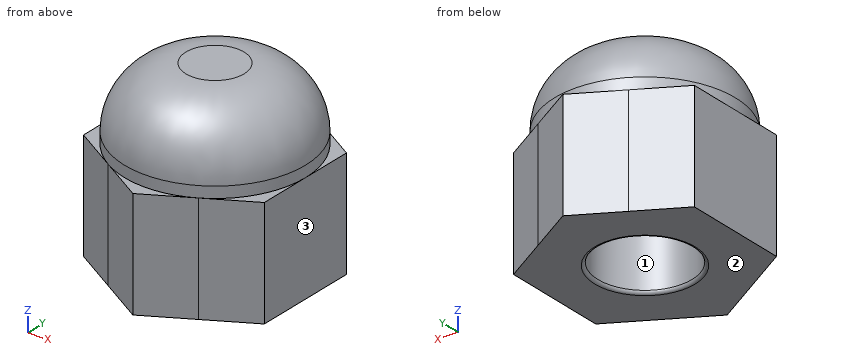
from build123d import *

# Parameters (mm, degrees)
SKETCH1_R           = 7.5
SKETCH1_R_2         = 3.9
BOSS_EXTRUDE1_DEPTH = 9
SKETCH2_R           = 7.5
BOSS_EXTRUDE2_DEPTH = 6
FILLET1_R           = 5.08
FILLET2_R           = 0.254


with BuildPart() as part:
    # Sketch1 → Boss-Extrude1 (new body)
    # profile 1 of 7: a face of its own
    with BuildSketch(Plane(origin=(0, 0, 0), x_dir=(0, 1, 0), z_dir=(0, 0, 1))):
        with BuildLine():
            ThreePointArc((-6.495190512, 3.750000029), (-3.749999976, 6.495190542), (2.2e-08, 7.5))
            Line((2.2e-08, 7.5), (-4.330127019, 7.5))
            Line((-4.330127019, 7.5), (-6.495190512, 3.750000029))
        make_face()
    # profile 2 of 7: a face of its own
    with BuildSketch(Plane(origin=(0, 0, 0), x_dir=(0, 1, 0), z_dir=(0, 0, 1))):
        Circle(SKETCH1_R)
        with Locations(Location((0, 0, 0), (0, 0, 270))):
            Circle(SKETCH1_R_2, mode=Mode.SUBTRACT)
    # profile 3 of 7: a face of its own
    with BuildSketch(Plane(origin=(0, 0, 0), x_dir=(0, 1, 0), z_dir=(0, 0, 1))):
        with BuildLine():
            ThreePointArc((2.2e-08, 7.5), (3.749999991, 6.495190533), (6.495190507, 3.750000037))
            Line((6.495190507, 3.750000037), (4.330127019, 7.5))
            Line((4.330127019, 7.5), (2.2e-08, 7.5))
        make_face()
    # profile 4 of 7: a face of its own
    with BuildSketch(Plane(origin=(0, 0, 0), x_dir=(0, 1, 0), z_dir=(0, 0, 1))):
        with BuildLine():
            ThreePointArc((-6.495190559, -3.749999947), (-7.5, 4.7e-08), (-6.495190512, 3.750000029))
            Line((-6.495190512, 3.750000029), (-8.660254038, 0))
            Line((-8.660254038, 0), (-6.495190559, -3.749999947))
        make_face()
    # profile 5 of 7: a face of its own
    with BuildSketch(Plane(origin=(0, 0, 0), x_dir=(0, 1, 0), z_dir=(0, 0, 1))):
        with BuildLine():
            Line((6.49519047, -3.750000102), (8.660254038, 0))
            Line((8.660254038, 0), (6.495190507, 3.750000037))
            ThreePointArc((6.495190507, 3.750000037), (7.244443692, 1.941142859), (7.5, 0))
            ThreePointArc((7.5, 0), (7.244443682, -1.941142895), (6.49519047, -3.750000102))
        make_face()
    # profile 6 of 7: a face of its own
    with BuildSketch(Plane(origin=(0, 0, 0), x_dir=(0, 1, 0), z_dir=(0, 0, 1))):
        with BuildLine():
            Line((4.330127019, -7.5), (6.49519047, -3.750000102))
            ThreePointArc((6.49519047, -3.750000102), (3.749999939, -6.495190564), (-2.3e-08, -7.5))
            Line((-2.3e-08, -7.5), (4.330127019, -7.5))
        make_face()
    # profile 7 of 7: a face of its own
    with BuildSketch(Plane(origin=(0, 0, 0), x_dir=(0, 1, 0), z_dir=(0, 0, 1))):
        with BuildLine():
            Line((-4.330127019, -7.5), (-2.3e-08, -7.5))
            ThreePointArc((-2.3e-08, -7.5), (-3.750000037, -6.495190507), (-6.495190559, -3.749999947))
            Line((-6.495190559, -3.749999947), (-4.330127019, -7.5))
        make_face()
    extrude(amount=BOSS_EXTRUDE1_DEPTH)

    # Sketch2 → Boss-Extrude2 (add)
    with BuildSketch(Plane.XY.offset(9)):
        Circle(SKETCH2_R)
    extrude(amount=BOSS_EXTRUDE2_DEPTH)

    # Fillet1
    fillet1_edges = [part.edges().sort_by_distance(p)[0] for p in [
        (-7.5, 0, 15),
    ]]
    fillet(fillet1_edges, radius=FILLET1_R)

    # Fillet2
    fillet2_edges = [part.edges().sort_by_distance(p)[0] for p in [
        (-3.9, 0, 0),
    ]]
    fillet(fillet2_edges, radius=FILLET2_R)


solid = part.part
Source: CAD feature listing. Evaluate the final solid. Frame: model axes, mm. Face numbers are marked on the shaded views. Coordinates: 2 decimals unless noted, no trailing zeros. Order: outer loops, then holes, each group sorted by start corner. A loop starts at its lowest first (then second) coordinate and runs counter-clockwise, first axis right, second up.
Item 1: Cut plane B-B (z = 9.5). Return loops of the section in (x, y).
Output values:
outline: circle Ø15 at (0, 0)
Item 2: First-contact query: P1, Ø6, axis at x = 0, y = 0, coming from the -Z side; P2, Ø1, axis at y = -6.5, z = 10.5, coming from the +X side; P3, Ø1, axis at x = 4.5, z = 9.5, coming from the -Y side. Flat tips, straight axial feed; report the tip coordinate or a pass-through.
Output values:
P1: stops at z = 9
P2: stops at x = 4.45
P3: stops at y = -6.34
Item 3: Cut plane A-A (z = 2.5). Return loops of the section in (x, y).
Output values:
outline: (-7.5, -4.33) - (0, -8.66) - (7.5, -4.33) - (7.5, 4.33) - (0, 8.66) - (-7.5, 4.33) - close; hole circle Ø7.8 at (0, 0)
Item 4: Material intervals for line 1 (Z direction, x = 1.5, y = -1.25); line 2 (Y direction, x = 2.5, z = 0.75); line 3 (X direction, y = 0.5, z = 3.5), sorted ascending.
Output values:
line 1: z = 9 to 15
line 2: y = -7.22 to -2.99, 2.99 to 7.22
line 3: x = -7.5 to -3.87, 3.87 to 7.5
Item 5: Pull-direction query (X, two-part tool) for the marked faces 1, 2 and 3; classes: pulls with the +X half, pulls with the -X half, needs draft (parallel to the pull), parting line crosses it, or undercut.
Output values:
face 1: undercut
face 2: needs draft
face 3: pulls with the +X half
